```python
from build123d import *

# Parameters (mm, degrees)
BOX042_W                                         = 10
BOX042_H                                         = 10
BOX042_DEPTH                                     = 5
BOX041_W                                         = 4
BOX041_H                                         = 14
BOX041_DEPTH                                     = 20
CHAMFER004013007011015006009007001005003019_SIZE = 3.5


with BuildPart() as cube042:
    # Box042 → Box042 (new body)
    with BuildSketch(Plane(origin=(-4.5, -5, 0), x_dir=(1, 0, 0), z_dir=(0, 0, 1))):
        with Locations((5, 5)):
            Rectangle(BOX042_W, BOX042_H)
    extrude(amount=BOX042_DEPTH)


with BuildPart() as block_remover_btm:
    # Box041 → Box041 (new body)
    with BuildSketch(Plane(origin=(-4.5, -7, 0), x_dir=(1, 0, 0), z_dir=(0, 0, 1))):
        with Locations((2, 7)):
            Rectangle(BOX041_W, BOX041_H)
    extrude(amount=BOX041_DEPTH)

    # Chamfer004013007011015006009007001005003019
    chamfer004013007011015006009007001005003019_edges = [block_remover_btm.edges().sort_by_distance(p)[0] for p in [
        (-0.5, -7, 10),
        (-0.5, 7, 10),
    ]]
    chamfer(chamfer004013007011015006009007001005003019_edges, length=CHAMFER004013007011015006009007001005003019_SIZE)

    # Fusion004025023011: union Cube042
    add(cube042.part)


solid = block_remover_btm.part
```
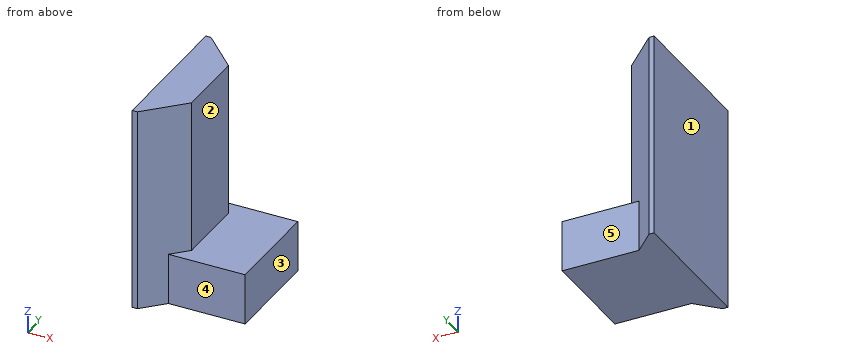
Geometry check sheet. Reference: the model listing, model coordinates, mm. Face numbers are marked on the shaded views. A direction names the side the tool comes from. Round coordinates to 2 decimals unless told otherwise and drop trailing zeros. Loops run counter-clockwise (first coordinate to the right, second up) from the corner with the lowest first, then second, coordinate; pieces in that order, holes last. Notation, with made-up numbers: (37, 3.25) - (80, 3.25) arc R12 ccw to (80, 21.25) - close; hole circle Ø2 at (1.25, 32). An arc over 180 degrees is marked (long way). Write each question's results on one line, items separated by ' | '. Start each with the question number.
Q1. Cross-section at B-B on x = -1.25. Enter the section's corners in (y, z).
Q2. Access from +Z, -Z, +X, -X, +Y, -Y to the whole of each face (thin tool, end or side, straight path). Record for the marked faces 1, 2, 3, 4 and 5.
Q3. Cross-section at C-C on y = 2.25. Enter the section's corners in (x, z), and give its area (3 significant figures).
Q4. Cross-section at A-A on z = 5.75. Enter the section's corners in (x, y), and give its area (4 significant figures).
Q5. Gauge pin test, flat ends, axial feed: P1, Ø4, axis at x = -1, z = 7.5, coming from the +Y side; P2, Ø2, axis at y = 0.5, z = 9, coming from the +X side; P3, Ø1.5, axis at x = -0.5, z = 7.5, coming from the +Y side. Record the tip position at first contact, or that the pin passes through.
Q6. Cross-section at D-D on z = 1. Enter the section's corners in (x, y).
Q7. Thickness scan on line 1 (X direction, y = 2.75, z = 7.5); line 2 (Z direction, x = 1, y = -1); line 3 (Y direction, x = 0, z = 1.5). Record the ranges inside material, lowest first. Write a range as [from, to].
Answers below:
1) outline: (-5, 0) - (5, 0) - (5, 5) - (4.25, 5) - (4.25, 20) - (-4.25, 20) - (-4.25, 5) - (-5, 5) - close
2) face 1: +Z, -Z, -X, +Y, -Y | face 2: +Z, +X, +Y, -Y | face 3: +Z, -Z, +X, +Y, -Y | face 4: +Z, -Z, +X, -Y | face 5: +Z, -Z, +X, +Y
3) outline: (-4.5, 0) - (5.5, 0) - (5.5, 5) - (-0.5, 5) - (-0.5, 20) - (-4.5, 20) - close | area: 110 mm²
4) outline: (-4.5, -7) - (-4, -7) - (-0.5, -3.5) - (-0.5, 3.5) - (-4, 7) - (-4.5, 7) - close | area: 43.75 mm²
5) P1: stops at y = 6 | P2: stops at x = -0.5 | P3: stops at y = 4.25
6) outline: (-4.5, -7) - (-4, -7) - (-2, -5) - (5.5, -5) - (5.5, 5) - (-2, 5) - (-4, 7) - (-4.5, 7) - close
7) line 1: x = [-4.5, -0.5] | line 2: z = [0, 5] | line 3: y = [-5, 5]
